Autodesk Inventor part; units mm, degrees
ref_plane "YZ Plane" through (0, 0, 0) normal (1, 0, 0) x (0, 1, 0)
ref_plane "XZ Plane" through (0, 0, 0) normal (0, 1, 0) x (-1, 0, 0)
ref_plane "XY Plane" through (0, 0, 0) normal (0, 0, 1) x (1, 0, 0)
sketch "Sketch1" plane through (0, 0, 0) normal (0, 0, 1) x (1, 0, 0)
  line L0 (-5, 5) -> (95, 5)
  line L1 (95, 5) -> (95, -5)
  line L2 (95, -5) -> (-5, -5)
  line L3 (-5, -5) -> (-5, 5)
  line L4 (0, 0) -> (0, 5) construction
  line L5 (0, 0) -> (0, -5) construction
  line L6 (0, 0) -> (-5, 0) construction
  dimension "d0" = 100
  dimension "d1" = 10
extrude "Extrusion1" add sketch "Sketch1" along normal blind 50
fillet "Fillet1" radius 3 2 edges at (-5, -5, 25) (-5, 5, 25)
sketch "Sketch2" plane through (0, 0, 50) normal (0, 0, 1) x (1, 0, 0)
  line L0 (2.0875, -1.55) -> (-2.0875, -1.55)
  line L1 (2.0875, 1.55) -> (-2.0875, 1.55)
  arc A0 (2.0875, -1.55) -> (2.0875, 1.55) centre (0, 0) ccw
  arc A1 (-2.0875, 1.55) -> (-2.0875, -1.55) centre (0, 0) ccw
  point P0 (2.6, 0)
  point P1 (-2.6, 0)
  dimension "d9" = 2.6
  dimension "d10" = 3.1
extrude "Extrusion2" cut sketch "Sketch2" against normal blind 8
sketch "Sketch3" plane through (0, 0, 50) normal (0, 0, 1) x (1, 0, 0)
  circle A0 centre (0, 0) radius 2.6
  dimension "d13" = 5.2
extrude "Extrusion3" cut sketch "Sketch3" against normal blind 1.5
properties part number "13042025-02"
Build history of the part. All positions in model axes, mm. A direction names the side the tool comes from. Round coordinates to 2 decimals unless told otherwise and drop trailing zeros. Write each loop counter-clockwise with the first axis right and the second up, starting at its lowest first coordinate (ties: lowest second). Pieces come first, ordered by that corner, then holes. Notation, with made-up numbers: (4.5, 8) - (50.5, 8) arc R30 cw to (50.5, 38) - close; hole circle Ø3 at (10.5, -5.75). An arc over 180 degrees is marked (long way). Write each question's results on one line, items separated by ' | '. Start each with the question number.
Item 1: Mould opens along X. For faces 3 (the face through (0, 0, 42)), 4 (the face through (47, -5, 25)), 5 (the face through (-4.1, 4.14, 25.35)) say: pulls with the +X half, pulls with the -X half, needs draft (parallel to the pull), parting line crosses it, or undercut.
Item 2: Which spindle directions (+Z, -Z, +X, -X, +Y, -Y) get a long thin tool onto all of the face, cutting with end or side? Do faces 1 (the face through (0, -1.55, 45)), 2 (the face through (-5, 0, 25)). Say none if no direction does.
Item 3: Saw through at A-A (z = 45). Write the cut outline in (x, y), and give its area (3 significant figures).
Item 4: Drop flat-ended pins along their axis: P1, Ø0.9, axis at x = 1, y = -0.5, coming from the +Z side; P2, Ø1.5, axis at y = -3.5, z = 28, coming from the -X side. Give the stop position or say it passes through.
Item 5: Wall check: L1, parallel to X at y = -2.25, z = 14.5; L2, parallel to X at y = 2.75, z = 47. Give the ranges that are in metal, low to high. Write a range as [from, to].
Results are:
1) face 3: undercut | face 4: needs draft | face 5: pulls with the -X half
2) face 1: +Z | face 2: +Z, -Z, -X, +Y, -Y
3) outline: (-5, -2) arc R3 ccw to (-2, -5) - (95, -5) - (95, 5) - (-2, 5) arc R3 ccw to (-5, 2) - close; hole (-2.09, -1.55) - (2.09, -1.55) arc R2.6 ccw to (2.09, 1.55) - (-2.09, 1.55) arc R2.6 ccw to start | area: 981 mm²
4) P1: stops at z = 42 | P2: stops at x = -4.9
5) L1: x = [-4.99, 95] | L2: x = [-4.9, 95]
